Can you work these out from the model? Positions are in its coordinate system, mm. A direction names the side the tool comes from. Round coordinates to 2 decimals unless told otherwise and drop trailing zeros. Loops run counter-clockwise (first coordinate to the right, second up) from the corner with the lowest first, then second, coordinate; pieces in that order, holes last.
Autodesk Inventor part; units mm, degrees
ref_plane "YZ Plane" through (0, 0, 0) normal (1, 0, 0) x (0, 1, 0)
ref_plane "XZ Plane" through (0, 0, 0) normal (0, 1, 0) x (-1, 0, 0)
ref_plane "XY Plane" through (0, 0, 0) normal (0, 0, 1) x (1, 0, 0)
sketch "Sketch1" plane through (0, 0, 0) normal (0, 1, 0) x (-1, 0, 0)
  line L0 (-6.35, 12.7) -> (6.35, 12.7)
  line L1 (6.35, 12.7) -> (6.35, -12.7)
  line L2 (6.35, -12.7) -> (-6.35, -12.7)
  line L3 (-6.35, -12.7) -> (-6.35, 12.7)
  line L4 (-6.35, 12.7) -> (6.35, -12.7) construction
  line L5 (6.35, 12.7) -> (-6.35, -12.7) construction
  line L6 (-9.525, 19.05) -> (9.525, 19.05)
  line L7 (9.525, 19.05) -> (9.525, -19.05)
  line L8 (9.525, -19.05) -> (-9.525, -19.05)
  line L9 (-9.525, -19.05) -> (-9.525, 19.05)
  line L10 (-9.525, 19.05) -> (9.525, -19.05) construction
  line L11 (9.525, 19.05) -> (-9.525, -19.05) construction
  line L12 (6.35, 15.875) -> (9.525, 15.875)
  line L13 (6.35, 15.875) -> (-9.525, 15.875)
  point P0 (0, 0)
  dimension "d0" = 12.7
  dimension "d1" = 25.4
extrude "Extrusion1" add sketch "Sketch1" along normal blind 3.175
sketch "Sketch2" plane through (0, 3.175, 0) normal (0, 1, 0) x (1, 0, 0)
  circle A0 centre (3.175, -9.525) radius 1.5875
  circle A1 centre (-3.175, 0) radius 1.5875
  circle A2 centre (0, 8.5298) radius 1.5
  line L0 (-4.318, -7.9375) -> (-2.032, -7.9375)
  line L1 (-2.032, -7.9375) -> (-2.032, -11.1125)
  line L2 (-2.032, -11.1125) -> (-4.318, -11.1125)
  line L3 (-4.318, -11.1125) -> (-4.318, -7.9375)
  line L4 (-4.318, -7.9375) -> (-2.032, -11.1125) construction
  line L5 (-2.032, -7.9375) -> (-4.318, -11.1125) construction
  line L6 (-9.525, 19.05) -> (-9.525, -19.05)
  line L7 (9.525, -19.05) -> (-9.525, -19.05)
  line L8 (-9.525, -19.05) -> (-9.525, 19.05)
  line L9 (-9.525, 19.05) -> (9.525, 19.05)
  line L10 (9.525, 19.05) -> (9.525, -19.05)
  line L11 (9.525, -19.05) -> (-9.525, 19.05) construction
  line L12 (-9.525, -19.05) -> (9.525, 19.05) construction
  point P0 (0, 0)
  point P1 (0, 0)
  dimension "d4" = 3.175
  dimension "d5" = 3.175
  dimension "d6" = 3
  dimension "d8" = 3.175
extrude "Extrusion2" add sketch "Sketch2" along normal blind 3.175
sketch "Sketch3" plane through (0, 6.35, 0) normal (0, 1, 0) x (1, 0, 0)
  line L0 (-9.525, 19.05) -> (-9.525, -19.05)
  line L1 (9.525, -19.05) -> (-9.525, -19.05)
  line L2 (-9.525, -19.05) -> (-9.525, 19.05)
  line L3 (-9.525, 19.05) -> (9.525, 19.05)
  line L4 (9.525, 19.05) -> (9.525, -19.05)
  line L5 (9.525, -19.05) -> (-9.525, 19.05) construction
  line L6 (-9.525, -19.05) -> (9.525, 19.05) construction
  line L7 (6.35, -12.7) -> (-6.35, -12.7)
  line L8 (-6.35, -12.7) -> (-6.35, 12.7)
  line L9 (-6.35, 12.7) -> (6.35, 12.7)
  line L10 (6.35, 12.7) -> (6.35, -12.7)
  line L11 (6.35, -12.7) -> (-6.35, 12.7) construction
  line L12 (-6.35, -12.7) -> (6.35, 12.7) construction
  point P0 (0, 0)
extrude "Extrusion3" add sketch "Sketch3" along normal blind 3.175
mirror "Mirror3" about plane through (-9.525, 0, 19.05) normal (0, 0, 1) of "Extrusion1", "Extrusion2", "Extrusion3"
properties part number "ExtendedSlottedCarrier"
(1) Suppose I cut it at C-C (y = 7.75). Write out the boundary of the cut face in (x, z) (3 decimals).
(2) For pin 1 (2 mm diameter, centred on x = -4.5, z = 42.5, fed in from +Y); pin 2 (1.9 mm diameter, centred on x = 3.175, z = 28.575, fed in from -Y); pin 3 (4 mm diameter, centred on x = -3.175, z = 38.1, fed in from -Y) (3 decimals), each with a flat end and sliding along its axis, tell me the tip position at first contact or that it passes through.
(3) Suppose I cut it at A-A (x = 0). Write out the boundary of the cut face in (y, z) (3 decimals), then the cut area to 3 significant figures.
(4) If I drill on line 1 (Z direction, x = -0.25, y = 2); line 2 (Z direction, x = 0, y = 4.1); line 3 (X direction, y = 2.5, z = 3) (3 decimals), over which ranges is the centre line in solid material (lowest first)?
(5) We'd pull the mould along X, two halves only. Please class faces 1 (the cylindrical face through (2.831, 4.74, 27.025)), 2 (the flat face through (0, 5, -19.05)): released by +X, released by -X, zero draft, split by the parting line, or undercut.
(6) Which directions (+Z, -Z, +X, -X, +Y, -Y) give clear straight access to the entire face, cutting with the end or side of a thin tool? Please do faces 3 (the flat face through (-3, 5, 11.112)), 4 (the flat face through (0, 9.525, 20)), 5 (the flat face through (0, 2, 12.7)), 6 (the flat face through (0, 6.35, 38)).
Check result:
1. outline: (-9.525, -19.05) - (9.525, -19.05) - (9.525, 57.15) - (-9.525, 57.15) - close; hole (-6.35, -12.7) - (6.35, -12.7) - (6.35, 12.7) - (-6.35, 12.7) - close; hole (-6.35, 25.4) - (6.35, 25.4) - (6.35, 50.8) - (-6.35, 50.8) - close
2. pin 1: stops at y = 6.35
2. pin 2: passes through
2. pin 3: stops at y = 3.175
3. outline: (0, -19.05) - (9.525, -19.05) - (9.525, -12.7) - (6.35, -12.7) - (6.35, -10.03) - (3.175, -10.03) - (3.175, -12.7) - (0, -12.7) - close; (0, 12.7) - (3.175, 12.7) - (3.175, -7.03) - (6.35, -7.03) - (6.35, 12.7) - (9.525, 12.7) - (9.525, 25.4) - (6.35, 25.4) - (6.35, 45.13) - (3.175, 45.13) - (3.175, 25.4) - (0, 25.4) - close; (0, 50.8) - (3.175, 50.8) - (3.175, 48.13) - (6.35, 48.13) - (6.35, 50.8) - (9.525, 50.8) - (9.525, 57.15) - (0, 57.15) - close
3. area: 384 mm2
4. line 1: z = -19.05 to -12.7, 12.7 to 25.4, 50.8 to 57.15
4. line 2: z = -19.05 to -10.03, -7.03 to 45.13, 48.13 to 57.15
4. line 3: x = -9.525 to -6.35, 6.35 to 9.525
5. face 1: undercut
5. face 2: zero draft
6. face 3: +Y, -Y
6. face 4: +Z, -Z, +X, -X, +Y
6. face 5: -Y
6. face 6: +Y
